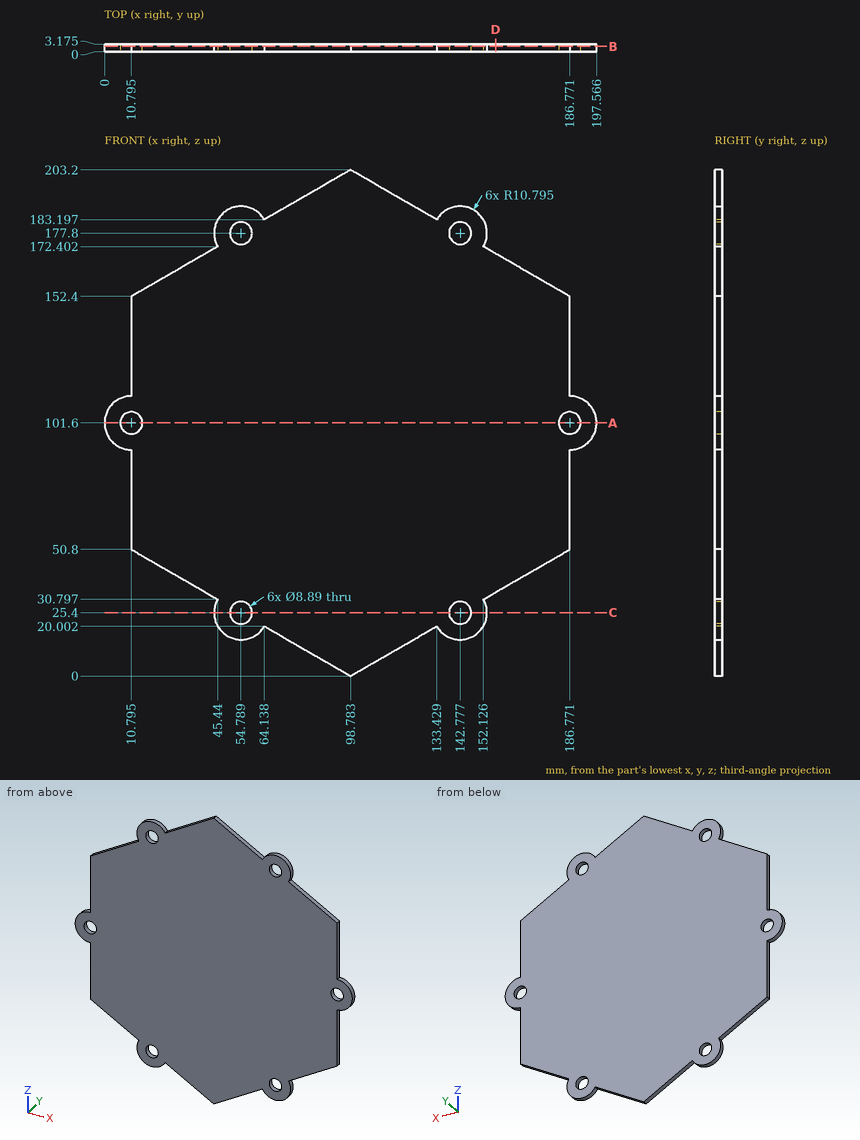
The drawing under review shows one solid part. Ordinate dimensions are in mm from its lowest x, y, z. Give positions to 0.01 mm unless a question says otherwise; leave off trailing zeros. Loops run counter-clockwise (first coordinate to the right, second up) from the corner with the lowest first, then second, coordinate; pieces in that order, holes last. Notation, with made-up numbers: M -29.5,-33 L 17.5,-33 A22 ccw 17.5,-23 Z; hole C 1.5,-19.5 d8. An arc over 180 degrees is marked long. One line per question, with ' | ' between items. Start each with the question number.
1. Add section D-D (x = 157). Write out the cut boundary in (y, z) (1 decimal).
2. Add section B-B (y = 2.2). Write out the cut boundary in (x, z) (1 decimal), plus the area to 3 significant figures.
3. Insertion check: P1, Ø7, axis at x = 54.79, z = 177.8, coming from the -Y side; P2, Ø1, axis at y = 2, z = 139.5, coming from the -X side (1 decimal); P3, Ø1.6, axis at y = 1, z = 70.5, coming from the +X side; P4, Ø1.5, axis at x = 141, y = 1.5, coming from the -Z side. Each pin has a flat end and moves straight along its axis. Give the tip position at first contact, or say it passes through.
4. Add section A-A (z = 101.6). Give the number of separate pieces and of enclosed holes in the cut face.
5. Add section C-C (z = 25.4). Write out the cut boundary in (x, y) (1 decimal).
6. To check wall thickness, follow L1, parallel to X at y = 0.45, z = 26 (1 decimal); L2, parallel to X at y = 1.6, z = 177.8 (1 decimal); L3, parallel to Z at x = 140, y = 0.3. State the ranges of each line that lie inside material, in increasing order.
Worked out:
1) outline: M 0,33.6 L 3.2,33.6 L 3.2,169.6 L 0,169.6 Z
2) outline: M 10.8,50.8 L 45.4,30.8 A10.8 ccw 64.1,20 L 98.8,0 L 133.4,20 A10.8 ccw 152.1,30.8 L 186.8,50.8 L 186.8,90.8 A10.8 ccw 186.8,112.4 L 186.8,152.4 L 152.1,172.4 A10.8 ccw 133.4,183.2 L 98.8,203.2 L 64.1,183.2 A10.8 ccw 45.4,172.4 L 10.8,152.4 L 10.8,112.4 A10.8 ccw 10.8,90.8 Z; hole C 10.8,101.6 d8.9; hole C 54.8,25.4 d8.9; hole C 54.8,177.8 d8.9; hole C 142.8,25.4 d8.9; hole C 142.8,177.8 d8.9; hole C 186.8,101.6 d8.9 | area: 27,500 mm²
3) P1: passes through | P2: stops at x = 10.8 | P3: stops at x = 186.77 | P4: stops at z = 14.65
4) separate pieces: 3 | enclosed holes: 0
5) outline: M 44,0 L 50.3,0 L 50.3,3.2 L 44,3.2 Z; M 59.2,0 L 138.3,0 L 138.3,3.2 L 59.2,3.2 Z; M 147.2,0 L 153.6,0 L 153.6,3.2 L 147.2,3.2 Z
6) L1: x = 44 to 50.4, 59.2 to 138.4, 147.2 to 153.6 | L2: x = 44 to 50.3, 59.2 to 138.3, 147.2 to 153.6 | L3: z = 14.97 to 21.93, 28.87 to 174.33, 181.27 to 188.23
